For this review, take the finished solid that the model builds, in its own axes (mm). A direction names the side the tool comes from. Give positions to 0.01 mm unless a question says otherwise; leave off trailing zeros. Write each loop counter-clockwise with the first axis right and the second up, starting at its lowest first coordinate (ties: lowest second). Pieces come first, ordered by that corner, then holes. Notation, with made-up numbers: M 22,32 L 52,32 A36 cw 52,66 Z; hole C -6,11 d1. An arc over 180 degrees is marked long. One line per item, written item: value. Start each with the question number.
Item 1: Tool access review of faces 4 (the face through (0, 34, -1)), 5 (the face through (0, 43, 0)), 6 (the face through (-1.73, -4.93, 7.81)): name each direction out of +Z, -Z, +X, -X, +Y, -Y from which nothing blocks a thin tool from reaching the whole face with its end or side.
Item 2: Consider section A-A, the plane z = 0. Write out the cut boundary in (x, y).
Item 3: Mouldability with a two-part tool opening along X and no side actions: class faces 1 (the face through (1.172, 12.325, -8.923)), 2 (the face through (-2, -10, -2)), 3 (the face through (0, -6, 0)) as released by +X, released by -X, zero draft, split by the parting line, or undercut.
Item 4: To check wall thickness, follow probe 1 along Z at (x, y) = (0, -8.65); probe 2 along Y at (x, z) = (5.25, 5); probe 3 along Z at (x, y) = (0.25, 17.5). State the ranges of each line that lie inside material, in increasing order.
Item 5: Consider section C-C, the plane x = -4.25. Write out the cut boundary in (y, z).
Item 6: Clearance check with flat-ended pins moving along their axes: pin 1 Ø4 at (y, z) = (12.5, -2.5) entering from -X; pin 2 Ø3 at (x, y) = (-1, 37) entering from +Z; pin 3 Ø3 at (x, y) = (-4, 18) entering from +Z; pin 4 Ø1 at (x, y) = (2, 29.5) entering from +Z. State where each tip first meets the part, or that it passes through.
Item 7: Consider section B-B, the plane x = 0. Write out the cut boundary in (y, z).
Item 8: Consider section D-D, the plane z = 3.75. Write out the cut boundary in (x, y), and give its area (3 significant figures).
Autodesk Inventor part; units mm, degrees
ref_plane "YZ Plane" through (0, 0, 0) normal (1, 0, 0) x (0, 1, 0)
ref_plane "XZ Plane" through (0, 0, 0) normal (0, 1, 0) x (-1, 0, 0)
ref_plane "XY Plane" through (0, 0, 0) normal (0, 0, 1) x (1, 0, 0)
sketch "Sketch1" plane through (0, 0, 0) normal (0, 1, 0) x (-1, 0, 0)
  circle A0 centre (0, 0) radius 10
  circle A1 centre (0, 0) radius 9
  dimension "d0" = 20
  dimension "d1" = 18
extrude "Extrusion1" add sketch "Sketch1" along normal blind 25 contours A1
sketch "Sketch2" plane through (0, 0, 0) normal (0, -1, 0) x (1, 0, 0)
  circle A0 centre (0, 0) radius 8
  dimension "d4" = 16
extrude "Extrusion2" add sketch "Sketch2" along normal blind 10
sketch "Sketch3" plane through (0, -10, 0) normal (0, -1, 0) x (1, 0, 0)
  circle A0 centre (0, 0) radius 2.5
  dimension "d7" = 5
extrude "Extrusion3" cut sketch "Sketch3" against normal blind 4
sketch "Sketch4" plane through (0, 25, 0) normal (0, 1, 0) x (1, 0, 0)
  circle A0 centre (0, 0) radius 1
  dimension "d10" = 2
extrude "Extrusion4" add sketch "Sketch4" along normal blind 18
sketch "Sketch5" plane through (0, -6, 0) normal (0, -1, 0) x (1, 0, 0)
  point P0 (0, 0)
properties part number "pump"
Model answer:
1. face 4: +Y
1. face 5: +Z, -Z, +X, -X, +Y
1. face 6: -Y
2. outline: M -9,0 L -8,0 L -8,-10 L -2.5,-10 L -2.5,-6 L 2.5,-6 L 2.5,-10 L 8,-10 L 8,0 L 9,0 L 9,25 L 1,25 L 1,43 L -1,43 L -1,25 L -9,25 Z
3. face 1: split by the parting line
3. face 2: zero draft
3. face 3: undercut
4. probe 1: z = -8 to -2.5, 2.5 to 8
4. probe 2: y = -10 to 25
4. probe 3: z = -9 to 9
5. outline: M -10,-6.78 L 0,-6.78 L 0,-7.93 L 25,-7.93 L 25,7.93 L 0,7.93 L 0,6.78 L -10,6.78 Z
6. pin 1: stops at x = -8.99
6. pin 2: stops at z = 1
6. pin 3: stops at z = 8.65
6. pin 4: passes through
7. outline: M -10,-8 L 0,-8 L 0,-9 L 25,-9 L 25,-1 L 43,-1 L 43,1 L 25,1 L 25,9 L 0,9 L 0,8 L -10,8 L -10,2.5 L -6,2.5 L -6,-2.5 L -10,-2.5 Z
8. outline: M -8.18,0 L -7.07,0 L -7.07,-10 L 7.07,-10 L 7.07,0 L 8.18,0 L 8.18,25 L -8.18,25 Z
8. area: 550 mm2
